from build123d import *

# Parameters (mm, degrees)
BOSS_EXTRUDE1_DEPTH = 3.175
FILLET1_R           = 80
FILLET2_R           = 8
SKETCH2_R           = 1.35
CUT_EXTRUDE1_DEPTH  = 136.741386774
SKETCH3_R           = 1.25
CUT_EXTRUDE2_DEPTH  = 136.741386774
SKETCH5_R           = 2.55
CUT_EXTRUDE3_DEPTH  = 136.741386774


with BuildPart() as part:
    # Sketch1 → Boss-Extrude1 (new body)
    with BuildSketch(Plane(origin=(0, 0, 0), x_dir=(1, 0, 0), z_dir=(0, 1, 0))):
        with BuildLine():
            Line((-70, 14), (-40, 14))
            Line((-40, 14), (-39.816062711, 70))
            Line((-39.816062711, 70), (-73.623466631, 79.058666579))
            ThreePointArc((-73.623466631, 79.058666579), (-83.522961568, 96.205094778), (-66.376533369, 106.104589715))
            Line((-66.376533369, 106.104589715), (0, 88.319051202))
            Line((0, 88.319051202), (66.376533369, 106.104589715))
            ThreePointArc((66.376533369, 106.104589715), (83.522961568, 96.205094778), (73.623466631, 79.058666579))
            Line((73.623466631, 79.058666579), (39.816062711, 70))
            Line((39.816062711, 70), (40, 14))
            Line((40, 14), (70, 14))
            ThreePointArc((70, 14), (84, 0), (70, -14))
            Line((70, -14), (40, -14))
            Line((40, -14), (39.816062711, -70))
            Line((39.816062711, -70), (73.623466631, -79.058666579))
            ThreePointArc((73.623466631, -79.058666579), (83.522961568, -96.205094778), (66.376533369, -106.104589715))
            Line((66.376533369, -106.104589715), (0, -88.319051202))
            Line((0, -88.319051202), (-66.376533369, -106.104589715))
            ThreePointArc((-66.376533369, -106.104589715), (-83.522961568, -96.205094778), (-73.623466631, -79.058666579))
            Line((-73.623466631, -79.058666579), (-39.816062711, -70))
            Line((-39.816062711, -70), (-40, -14))
            Line((-40, -14), (-70, -14))
            ThreePointArc((-70, -14), (-84, 0), (-70, 14))
        make_face()
    extrude(amount=BOSS_EXTRUDE1_DEPTH)

    # Fillet1
    fillet1_edges = [part.edges().sort_by_distance(p)[0] for p in [
        (0, 1.5875, -88.319051202),
        (0, 1.5875, 88.319051202),
    ]]
    fillet(fillet1_edges, radius=FILLET1_R)

    # Fillet2
    fillet2_edges = [part.edges().sort_by_distance(p)[0] for p in [
        (-40, 1.5875, -14),
        (-39.816062711, 1.5875, -70),
        (39.816062711, 1.5875, -70),
        (40, 1.5875, -14),
        (40, 1.5875, 14),
        (39.816062711, 1.5875, 70),
        (-39.816062711, 1.5875, 70),
        (-40, 1.5875, 14),
    ]]
    fillet(fillet2_edges, radius=FILLET2_R)

    # Sketch2 → Cut-Extrude1 (cut, through all)
    with BuildSketch(Plane(origin=(0, 3.175, 0), x_dir=(1, 0, 0), z_dir=(0, 1, 0))):
        with Locations(Location((-24.5, 24.641145635, 0), (0, 0, 270))):
            Circle(SKETCH2_R)
        with Locations(Location((24.5, 24.641145635, 0), (0, 0, 270))):
            Circle(SKETCH2_R)
        with Locations(Location((24.5, 82.641145635, 0), (0, 0, 270))):
            Circle(SKETCH2_R)
        with Locations(Location((-24.5, 82.641145635, 0), (0, 0, 270))):
            Circle(SKETCH2_R)
    extrude(amount=-CUT_EXTRUDE1_DEPTH, mode=Mode.SUBTRACT)

    # Sketch3 → Cut-Extrude2 (cut, through all)
    with BuildSketch(Plane(origin=(0, 3.175, 0), x_dir=(1, 0, 0), z_dir=(0, 1, 0))):
        with Locations(Location((-8.3, -40.058854365, 0), (0, 0, 270))):
            Circle(SKETCH3_R)
        with Locations(Location((-27.1, -40.058854365, 0), (0, 0, 270))):
            Circle(SKETCH3_R)
        with Locations(Location((-27.1, 15.841145635, 0), (0, 0, 270))):
            Circle(SKETCH3_R)
        with Locations(Location((-8.3, 15.841145635, 0), (0, 0, 270))):
            Circle(SKETCH3_R)
        with Locations(Location((8.3, 15.841145635, 0), (0, 0, 270))):
            Circle(SKETCH3_R)
        with Locations(Location((27.1, 15.841145635, 0), (0, 0, 270))):
            Circle(SKETCH3_R)
        with Locations(Location((8.3, -40.058854365, 0), (0, 0, 270))):
            Circle(SKETCH3_R)
        with Locations(Location((27.1, -40.058854365, 0), (0, 0, 270))):
            Circle(SKETCH3_R)
    extrude(amount=-CUT_EXTRUDE2_DEPTH, mode=Mode.SUBTRACT)

    # Sketch5 → Cut-Extrude3 (cut, through all)
    with BuildSketch(Plane(origin=(0, 3.175, 0), x_dir=(1, 0, 0), z_dir=(0, 1, 0))):
        with Locations(Location((0, -56.018854365, 0), (0, 0, 270))):
            Circle(SKETCH5_R)
    extrude(amount=-CUT_EXTRUDE3_DEPTH, mode=Mode.SUBTRACT)


solid = part.part
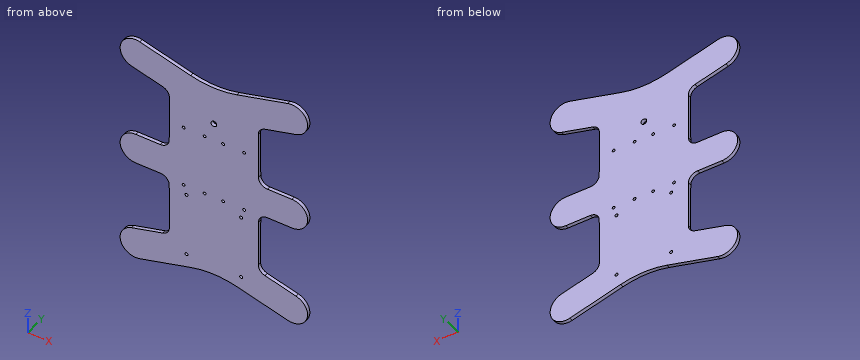
Geometry check sheet. Reference: the model listing, model coordinates, mm. Round coordinates to 2 decimals unless told otherwise and drop trailing zeros. Loops run counter-clockwise (first coordinate to the right, second up) from the corner with the lowest first, then second, coordinate; pieces in that order, holes last.
Item 1: Cross-section at D-D on z = -76.5. Record the boundary of the cut face in (x, y) (3 decimals).
Item 2: Cross-section at B-B on x = -58. Record the boundary of the cut face in (y, z) (3 decimals), then the cut area to 3 significant figures.
Item 3: Cross-section at C-C on y = 0.9. Count the separate pieces of the cut face and the enclosed holes in it, then the cut area to 3 significant figures.
Item 4: Gauge pin test, flat ends, axial feed: pin 1 (3.5 mm diameter, centred on x = -24.5, z = -82.64, fed in from +Y) (3 decimals); pin 2 (1 mm diameter, centred on x = -55, y = 1.5, fed in from +Z); pin 3 (1.6 mm diameter, centred on x = 24.5, z = -24.64, fed in from +Y); pin 4 (1.5 mm diameter, centred on x = -31, y = 2, fed in from +Z). Record the tip position at first contact, or that the pin passes through.
Item 5: Thickness scan on line 1 (X direction, y = 2.25, z = -25); line 2 (Z direction, x = 8.5, y = 2); line 3 (Z direction, x = 57, y = 2.7). Record the ranges inside material, lowest first.
Item 6: Cross-section at A-A on x = 0. Record the boundary of the cut face in (y, z) (3 decimals), then the cut area to 3 significant figures.
Answer sheet:
1. outline: (-64.074, 0) - (64.074, 0) - (64.074, 3.175) - (-64.074, 3.175) - close
2. outline: (0, -103.86) - (3.175, -103.86) - (3.175, -74.872) - (0, -74.872) - close; (0, -14) - (3.175, -14) - (3.175, 14) - (0, 14) - close; (0, 74.872) - (3.175, 74.872) - (3.175, 103.86) - (0, 103.86) - close
2. area: 273 mm2
3. separate pieces: 1
3. enclosed holes: 13
3. area: 22,100 mm2
4. pin 1: stops at y = 3.175
4. pin 2: stops at z = 103.19
4. pin 3: passes through
4. pin 4: stops at z = 96.83
5. line 1: x = -39.96 to -25.8, -23.2 to 23.2, 25.8 to 39.96
5. line 2: z = -91.59 to -17.08, -14.61 to 38.82, 41.29 to 91.59
5. line 3: z = -103.59 to -74.6, -14 to 14, 74.6 to 103.59
6. outline: (0, -91.141) - (3.175, -91.141) - (3.175, 53.469) - (0, 53.469) - close; (0, 58.569) - (3.175, 58.569) - (3.175, 91.141) - (0, 91.141) - close
6. area: 563 mm2
